Geometry: final body of the model. Coordinates: model frame, mm. Give positions to 0.01 mm unless a question says otherwise; leave off trailing zeros. Order: outer loops, then holes, each group sorted by start corner. A loop starts at its lowest first (then second) coordinate and runs counter-clockwise, first axis right, second up. Notation, with made-up numbers: (17, 34.5) -> (65, 34.5) arc R33 cw to (65, 68.5) -> close; hole circle Ø5 at (30, 87.25). An arc over 180 degrees is marked (long way). One line per item, written item: value. Start each with the question number.
```python
from build123d import *

# Parameters (mm, degrees)
SKETCH1_R           = 5.05
SKETCH1_R_2         = 2.51
SKETCH1_R_3         = 2.5
SKETCH1_W           = 2.75
SKETCH1_H           = 6.7
BOSS_EXTRUDE1_DEPTH = 6.35
SKETCH1_4_W         = 2.75
SKETCH1_4_H         = 6.7
CUT_EXTRUDE1_DEPTH  = 2.18
SKETCH1_5_R         = 5.05
SKETCH1_5_R_2       = 2.5
CUT_EXTRUDE2_DEPTH  = 2


with BuildPart() as part:
    # Sketch1 → Boss-Extrude1 (new body)
    # profile 1 of 7: a face of its own
    with BuildSketch(Plane(origin=(0, 0, 0), x_dir=(1, 0, 0), z_dir=(0, 1, 0))):
        with BuildLine():
            ThreePointArc((0, 6.17), (1.80715116, 1.80715116), (6.17, 0))
            Line((6.17, 0), (43.83, 0))
            ThreePointArc((43.83, 0), (48.19284884, 1.80715116), (50, 6.17))
            Line((50, 6.17), (50, 21.65))
            Line((50, 21.65), (47.25, 21.65))
            Line((47.25, 21.65), (44.75, 21.65))
            Line((44.75, 21.65), (44.75, 28.35))
            Line((44.75, 28.35), (47.25, 28.35))
            Line((47.25, 28.35), (50, 28.35))
            Line((50, 28.35), (50, 43.83))
            ThreePointArc((50, 43.83), (48.19284884, 48.19284884), (43.83, 50))
            Line((43.83, 50), (6.17, 50))
            ThreePointArc((6.17, 50), (1.80715116, 48.19284884), (0, 43.83))
            Line((0, 43.83), (0, 28.35))
            Line((0, 28.35), (2.75, 28.35))
            Line((2.75, 28.35), (5.25, 28.35))
            Line((5.25, 28.35), (5.25, 21.65))
            Line((5.25, 21.65), (2.75, 21.65))
            Line((2.75, 21.65), (0, 21.65))
            Line((0, 21.65), (0, 6.17))
        make_face()
        with Locations((10, 9.05)):
            Circle(SKETCH1_R, mode=Mode.SUBTRACT)
        with Locations((40, 9.05)):
            Circle(SKETCH1_R, mode=Mode.SUBTRACT)
        with Locations(Location((25, 15, 0), (0, 0, 270))):
            Circle(SKETCH1_R_2, mode=Mode.SUBTRACT)
        with Locations(Location((15, 25, 0), (0, 0, 270))):
            Circle(SKETCH1_R_2, mode=Mode.SUBTRACT)
        with Locations((10, 40.95)):
            Circle(SKETCH1_R, mode=Mode.SUBTRACT)
        with Locations(Location((25, 25, 0), (0, 0, 270))):
            Circle(SKETCH1_R_2, mode=Mode.SUBTRACT)
        with Locations(Location((35, 25, 0), (0, 0, 270))):
            Circle(SKETCH1_R_2, mode=Mode.SUBTRACT)
        with Locations(Location((25, 35, 0), (0, 0, 270))):
            Circle(SKETCH1_R_2, mode=Mode.SUBTRACT)
        with Locations((40, 40.95)):
            Circle(SKETCH1_R, mode=Mode.SUBTRACT)
    # profile 2 of 7: a face of its own
    with BuildSketch(Plane(origin=(0, 0, 0), x_dir=(1, 0, 0), z_dir=(0, 1, 0))):
        with Locations((40, 40.95)):
            Circle(SKETCH1_R)
        with Locations(Location((40, 40.95, 0), (0, 0, 270))):
            Circle(SKETCH1_R_3, mode=Mode.SUBTRACT)
    # profile 3 of 7: a face of its own
    with BuildSketch(Plane(origin=(0, 0, 0), x_dir=(1, 0, 0), z_dir=(0, 1, 0))):
        with Locations((48.625, 25)):
            Rectangle(SKETCH1_W, SKETCH1_H)
    # profile 4 of 7: a face of its own
    with BuildSketch(Plane(origin=(0, 0, 0), x_dir=(1, 0, 0), z_dir=(0, 1, 0))):
        with Locations((40, 9.05)):
            Circle(SKETCH1_R)
        with Locations(Location((40, 9.05, 0), (0, 0, 270))):
            Circle(SKETCH1_R_3, mode=Mode.SUBTRACT)
    # profile 5 of 7: a face of its own
    with BuildSketch(Plane(origin=(0, 0, 0), x_dir=(1, 0, 0), z_dir=(0, 1, 0))):
        with Locations((10, 9.05)):
            Circle(SKETCH1_R)
        with Locations(Location((10, 9.05, 0), (0, 0, 270))):
            Circle(SKETCH1_R_3, mode=Mode.SUBTRACT)
    # profile 6 of 7: a face of its own
    with BuildSketch(Plane(origin=(0, 0, 0), x_dir=(1, 0, 0), z_dir=(0, 1, 0))):
        with Locations((10, 40.95)):
            Circle(SKETCH1_R)
        with Locations(Location((10, 40.95, 0), (0, 0, 270))):
            Circle(SKETCH1_R_3, mode=Mode.SUBTRACT)
    # profile 7 of 7: a face of its own
    with BuildSketch(Plane(origin=(0, 0, 0), x_dir=(1, 0, 0), z_dir=(0, 1, 0))):
        with Locations((1.375, 25)):
            Rectangle(SKETCH1_W, SKETCH1_H)
    extrude(amount=-BOSS_EXTRUDE1_DEPTH)

    # Sketch1_4 → Cut-Extrude1 (cut)
    with BuildSketch(Plane(origin=(0, 0, 0), x_dir=(1, 0, 0), z_dir=(0, 1, 0))):
        with Locations((1.375, 25)):
            Rectangle(SKETCH1_4_W, SKETCH1_4_H)
        with Locations((48.625, 25)):
            Rectangle(SKETCH1_4_W, SKETCH1_4_H)
    extrude(amount=-CUT_EXTRUDE1_DEPTH, mode=Mode.SUBTRACT)

    # Sketch1_5 → Cut-Extrude2 (cut)
    # profile 1 of 4: a face of its own
    with BuildSketch(Plane(origin=(0, 0, 0), x_dir=(1, 0, 0), z_dir=(0, 1, 0))):
        with Locations(Location((10, 40.95, 0), (0, 0, 270))):
            Circle(SKETCH1_5_R)
        with Locations(Location((10, 40.95, 0), (0, 0, 270))):
            Circle(SKETCH1_5_R_2, mode=Mode.SUBTRACT)
    # profile 2 of 4: a face of its own
    with BuildSketch(Plane(origin=(0, 0, 0), x_dir=(1, 0, 0), z_dir=(0, 1, 0))):
        with Locations(Location((40, 40.95, 0), (0, 0, 270))):
            Circle(SKETCH1_5_R)
        with Locations(Location((40, 40.95, 0), (0, 0, 270))):
            Circle(SKETCH1_5_R_2, mode=Mode.SUBTRACT)
    # profile 3 of 4: a face of its own
    with BuildSketch(Plane(origin=(0, 0, 0), x_dir=(1, 0, 0), z_dir=(0, 1, 0))):
        with Locations(Location((40, 9.05, 0), (0, 0, 270))):
            Circle(SKETCH1_5_R)
        with Locations(Location((40, 9.05, 0), (0, 0, 270))):
            Circle(SKETCH1_5_R_2, mode=Mode.SUBTRACT)
    # profile 4 of 4: a face of its own
    with BuildSketch(Plane(origin=(0, 0, 0), x_dir=(1, 0, 0), z_dir=(0, 1, 0))):
        with Locations(Location((10, 9.05, 0), (0, 0, 270))):
            Circle(SKETCH1_5_R)
        with Locations(Location((10, 9.05, 0), (0, 0, 270))):
            Circle(SKETCH1_5_R_2, mode=Mode.SUBTRACT)
    extrude(amount=-CUT_EXTRUDE2_DEPTH, mode=Mode.SUBTRACT)


solid = part.part
```
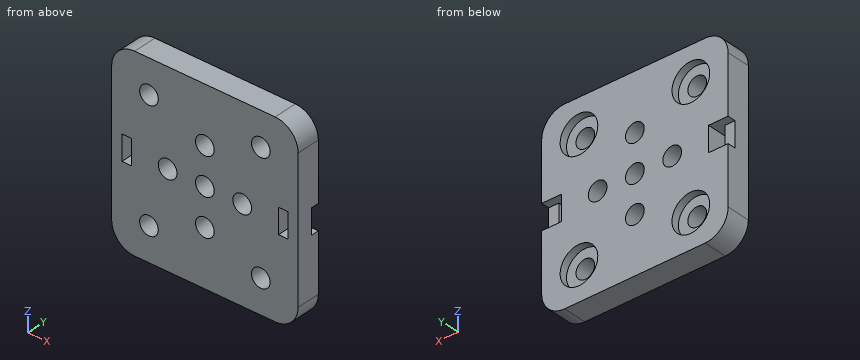
1. Cut plane B-B, the plane z = -15. Return loops of the section in (x, y), then the cut area to 3 significant figures.
2. Cut plane C-C, the plane y = -5.5. State how many separate pieces and enclosed holes the cut face has, then the cut area to 3 significant figures.
3. Cut plane D-D, the plane z = -40.95. Return loops of the section in (x, y), then the cut area to 3 significant figures.
4. Pin query (flat end, axial travel): P1, Ø6, axis at x = 25, z = -15, coming from the -Y side; P2, Ø3, axis at x = 9, z = -38.5, coming from the +Y side; P3, Ø1.4, axis at x = 48.5, z = -26, coming from the +Y side; P4, Ø1.6, axis at x = 47, y = -4.5, coming from the -Z side. Return the tip coordinate at first contact, or that it passes through.
5. Material intervals for L1, parallel to X at y = -3.75, z = -25; L2, parallel to X at y = -4.9, z = -9.05; L3, parallel to X at y = -0.7, z = -40.95, sorted ascending. Write a range as [from, to].
6. Cut plane A-A, the plane x = 40. Return loops of the section in (y, z).
Answers follow:
1. outline: (0, -6.35) -> (22.49, -6.35) -> (22.49, 0) -> (0, 0) -> close; (27.51, -6.35) -> (50, -6.35) -> (50, 0) -> (27.51, 0) -> close
1. area: 286 mm²
2. separate pieces: 1
2. enclosed holes: 11
2. area: 2,260 mm²
3. outline: (0, -6.35) -> (7.5, -6.35) -> (7.5, -2) -> (4.95, -2) -> (4.95, 0) -> (0, 0) -> close; (12.5, -6.35) -> (37.5, -6.35) -> (37.5, -2) -> (34.95, -2) -> (34.95, 0) -> (15.05, 0) -> (15.05, -2) -> (12.5, -2) -> close; (42.5, -6.35) -> (50, -6.35) -> (50, 0) -> (45.05, 0) -> (45.05, -2) -> (42.5, -2) -> close
3. area: 234 mm²
4. P1: stops at y = -6.35
4. P2: stops at y = -2
4. P3: stops at y = -2.18
4. P4: stops at z = -49.53
5. L1: x = [0, 2.75], [5.25, 12.49], [17.51, 22.49], [27.51, 32.49], [37.51, 44.75], [47.25, 50]
5. L2: x = [0, 7.5], [12.5, 37.5], [42.5, 50]
5. L3: x = [0, 4.95], [15.05, 34.95], [45.05, 50]
6. outline: (-6.35, -50) -> (0, -50) -> (0, -46) -> (-2, -46) -> (-2, -43.45) -> (-6.35, -43.45) -> close; (-6.35, -38.45) -> (-2, -38.45) -> (-2, -35.9) -> (0, -35.9) -> (0, -14.1) -> (-2, -14.1) -> (-2, -11.55) -> (-6.35, -11.55) -> close; (-6.35, -6.55) -> (-2, -6.55) -> (-2, -4) -> (0, -4) -> (0, 0) -> (-6.35, 0) -> close
